For this review, take the finished solid that the model builds, in its own axes (mm). Face numbers are marked on the shaded views. A direction names the side the tool comes from. Round coordinates to 2 decimals unless told otherwise and drop trailing zeros. Loops run counter-clockwise (first coordinate to the right, second up) from the corner with the lowest first, then second, coordinate; pieces in that order, holes last. Notation, with made-up numbers: (-30.75, 64) -> (23.25, 64) arc R16 ccw to (23.25, 76) -> close; hole circle Ø1 at (71, 28.25). An arc over 180 degrees is marked (long way). Write each question's results on one line, items separated by ' | '.
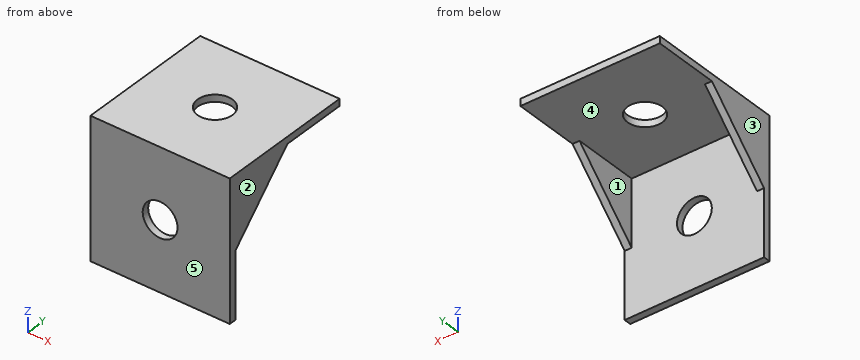
```python
from build123d import *

# Parameters (mm, degrees)
SKETCH1_W           = 20
SKETCH1_H           = 20
SKETCH1_R           = 2.5
BOSS_EXTRUDE1_DEPTH = 1
SKETCH2_W           = 20
SKETCH2_H           = 20
SKETCH2_R           = 2.5
BOSS_EXTRUDE2_DEPTH = 1
BOSS_EXTRUDE3_DEPTH = 1
BOSS_EXTRUDE4_START = -19
BOSS_EXTRUDE4_DEPTH = 1


with BuildPart() as part:
    # Sketch1 → Boss-Extrude1 (new body)
    with BuildSketch(Plane(origin=(0, 0, 0), x_dir=(1, 0, 0), z_dir=(0, 1, 0))):
        Rectangle(SKETCH1_W, SKETCH1_H)
        with Locations(Location((0, 0, 0), (0, 0, 270))):
            Circle(SKETCH1_R, mode=Mode.SUBTRACT)
    extrude(amount=BOSS_EXTRUDE1_DEPTH)

    # Sketch2 → Boss-Extrude2 (add)
    with BuildSketch(Plane.XY.offset(10)):
        with Locations((0, 10)):
            Rectangle(SKETCH2_W, SKETCH2_H)
        with Locations((0, 10)):
            Circle(SKETCH2_R, mode=Mode.SUBTRACT)
    extrude(amount=-BOSS_EXTRUDE2_DEPTH)

    # Sketch3 → Boss-Extrude3 (add)
    with BuildSketch(Plane(origin=(10, 0, 0), x_dir=(0, 0, -1), z_dir=(1, 0, 0))):
        Polygon((-9, 10.5), (0.5, 1), (-9, 1), align=None)
    extrude(amount=-BOSS_EXTRUDE3_DEPTH)

    # Sketch3_2 → Boss-Extrude4 (add)
    with BuildSketch(Plane(origin=(10, 0, 0), x_dir=(0, 0, -1), z_dir=(1, 0, 0)).offset(BOSS_EXTRUDE4_START)):
        Polygon((-9, 10.5), (0.5, 1), (-9, 1), align=None)
    extrude(amount=-BOSS_EXTRUDE4_DEPTH)


solid = part.part
```
1. Consider section A-A (z = 0). State the section outline as (x, y) points.
Values found:
outline: (-10, 0) -> (-2.5, 0) -> (-2.5, 1) -> (-9, 1) -> (-9, 1.5) -> (-10, 1.5) -> close; (2.5, 0) -> (10, 0) -> (10, 1.5) -> (9, 1.5) -> (9, 1) -> (2.5, 1) -> close
2. For pin 1 (3 mm diameter, centred on x = 0, z = 0, fed in from -Y); pin 2 (8 mm diameter, centred on x = 0.5, y = 7.5, fed in from -Z); pin 3 (5.5 mm diameter, centred on x = -1, z = -5, fed in from +Y), all flat-tipped, find the tip position at first contact; note any pin that passes through.
Values found:
pin 1: passes through | pin 2: stops at z = 9 | pin 3: stops at y = 1
3. Consider section C-C (y = 10). State the section outline as (x, z) points.
Values found:
outline: (-10, 8.5) -> (-9, 8.5) -> (-9, 9) -> (-2.5, 9) -> (-2.5, 10) -> (-10, 10) -> close; (2.5, 9) -> (9, 9) -> (9, 8.5) -> (10, 8.5) -> (10, 10) -> (2.5, 10) -> close
4. Consider section D-D (z = 5.25). State the section outline as (x, y) points, plus the area to 3 significant figures.
Values found:
outline: (-10, 0) -> (10, 0) -> (10, 6.75) -> (9, 6.75) -> (9, 1) -> (-9, 1) -> (-9, 6.75) -> (-10, 6.75) -> close | area: 31.5 mm2
5. Draft analysis for pull direction X (two halves, no side actions). For the marked faces 3, 4 and 5, state which applies: released by +X, released by -X, zero draft, split by the parting line, or undercut.
Values found:
face 3: released by -X | face 4: undercut | face 5: zero draft
6. Tool access review of the marked faces 1 and 2: name each direction out of +Z, -Z, +X, -X, +Y, -Y from which nothing blocks a thin tool from reaching the whole face with its end or side.
Values found:
face 1: -Z, +Y | face 2: +Z, -Z, +X, +Y, -Y
7. To check wall thickness, follow probe 1 along X at (y, z) = (0.3, 0); probe 2 along Y at (x, z) = (0, 9.5); probe 3 along X at (y, z) = (7, 7). State the ranges of each line that lie inside material, in increasing order.
Values found:
probe 1: x = -10 to -2.5, 2.5 to 10 | probe 2: y = 0 to 7.5, 12.5 to 20 | probe 3: x = -10 to -9, 9 to 10
8. Consider section B-B (x = 0). State the section outline as (y, z) points.
Values found:
outline: (0, -10) -> (1, -10) -> (1, -2.5) -> (0, -2.5) -> close; (0, 2.5) -> (1, 2.5) -> (1, 9) -> (7.5, 9) -> (7.5, 10) -> (0, 10) -> close; (12.5, 9) -> (20, 9) -> (20, 10) -> (12.5, 10) -> close
